Input: dimensioned drawing with shaded views. Units: mm. Origin: part minimum x, y, z. Give positions to 0.01 mm unless a question says otherwise; leave off trailing zeros. Write each loop counter-clockwise with the first axis right and the second up, starting at its lowest first coordinate (ties: lowest second). Pieces come first, ordered by that corner, then holes.
Q1. Pin query (flat end, axial travel): pin 1 Ø5 at (x, z) = (77.08, 24.92) entering from +Y; pin 2 Ø2.5 at (x, z) = (2.92, 24.92) entering from +Y. Return the tip coordinate at first contact, or that it passes through.
Q2. Line query: line 1 (X direction, y = 0.55, z = 77); line 2 (Z direction, x = 55.5, y = 0.15); line 3 (X direction, y = 1.9, z = 76.5). Output: solid intervals per line, ascending.
Q3. Section A-A (z = 77). Return the cut outline in (x, y), plus the area to 3 significant figures.
Q4. Section B-B (x = 25). Return the cut outline in (y, z), plus the area to 3 significant figures.
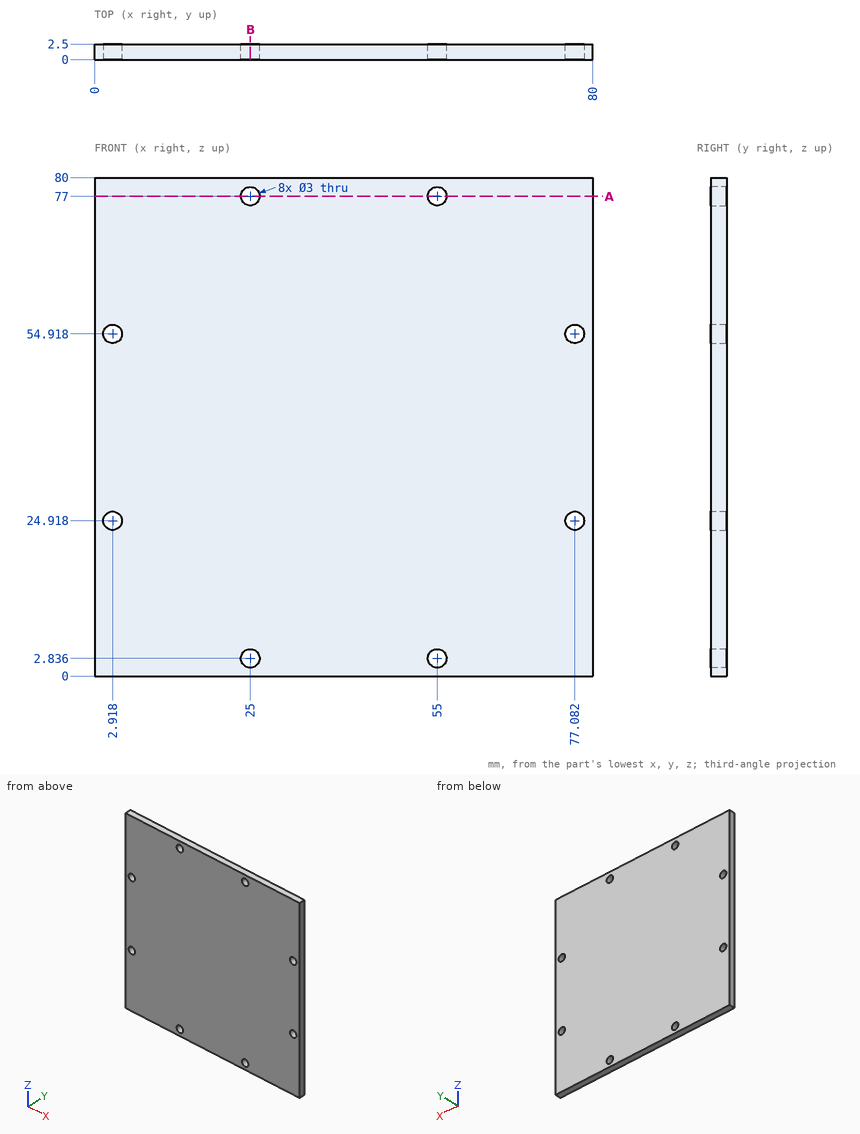
Computed:
1. pin 1: stops at y = 2.5
1. pin 2: passes through
2. line 1: x = 0 to 23.5, 26.5 to 53.5, 56.5 to 80
2. line 2: z = 0 to 1.42, 4.25 to 75.59, 78.41 to 80
2. line 3: x = 0 to 23.59, 26.41 to 53.59, 56.41 to 80
3. outline: (0, 0) - (23.5, 0) - (23.5, 2.5) - (0, 2.5) - close; (26.5, 0) - (53.5, 0) - (53.5, 2.5) - (26.5, 2.5) - close; (56.5, 0) - (80, 0) - (80, 2.5) - (56.5, 2.5) - close
3. area: 185 mm2
4. outline: (0, 0) - (2.5, 0) - (2.5, 1.34) - (0, 1.34) - close; (0, 4.34) - (2.5, 4.34) - (2.5, 75.5) - (0, 75.5) - close; (0, 78.5) - (2.5, 78.5) - (2.5, 80) - (0, 80) - close
4. area: 185 mm2
